Check sheet for the modelled part. Datum: model origin and axes. Units: mm. A direction names the side the tool comes from. Give positions to 0.01 mm unless a question says otherwise; leave off trailing zeros. Use a Markdown table: item, result. Add a question column.
1. Gauge pin test, flat ends, axial feed: P1, Ø4, axis at x = -4.195, z = 1.04, coming from the -Y side; P2, Ø0.5, axis at x = 4, z = 1, coming from the -Y side; P3, Ø0.5, axis at x = -4, z = 1, coming from the -Y side. Record the tip position at first contact, or that the pin passes through.
2. Release check for a two-part mould opening along X. For faces 1 (the cylindrical face through (-8.565, 6.83, 5.449)), 2 (the flat face through (0, 7, -5.75)), 3 (the flat face through (4, 4, 1)) record: released by +X, released by -X, zero draft, split by the parting line, or undercut.
3. Cross-section at A-A (y = 1.5). Count the separate pieces of the cut face and the enclosed holes in it, then the cut area to 3 significant figures.
4. Scan lines: probe 1 along X at (y, z) = (0.8, 1.04) (3 decimals); probe 2 along X at (y, z) = (0.5, 1.04) (3 decimals); probe 3 along Y at (x, z) = (4.5, 0.75). Record each from-to range of solid material in increasing order. Write a range as [from, to].
5. Set-up check for faces 4 (the cylindrical face through (2.21, 0.99, -0.48)), 5 (the cylindrical face through (-8.565, 0.301, 0.067)): record each of +Z, -Z, +X, -X, +Y, -Y from which the full face is reachable in a straight line by a thin tool's end or side.
Autodesk Fusion 360 part; units mm, degrees
sketch "Boceto1" plane through (0, 0, 0) normal (0, 1, 0) x (1, 0, 0)
  line L0 (-8.85, 0) -> (-8.85, -5.75)
  line L1 (-8.85, -5.75) -> (8.85, -5.75)
  line L2 (8.85, -5.75) -> (8.85, 5.75)
  line L3 (8.85, 5.75) -> (-8.85, 5.75)
  line L4 (-8.85, 5.75) -> (-8.85, 0)
  dimension "d1" = 8.85
  dimension "d2" = 5.75
  dimension "d3" = 17.7
  dimension "d4" = 11.5
  dimension "d5" = 17.7
extrude "Extruir1" add sketch "Boceto1" along normal blind 12.5
sketch "Boceto2" plane through (0, 0, 0) normal (0, -1, 0) x (1, 0, 0)
  line L0 (-8.85, 5.75) -> (-8.85, -5.75)
  line L1 (-8.85, -5.75) -> (8.85, -5.75)
  line L2 (8.85, -5.75) -> (8.85, 5.75)
  line L3 (8.85, 5.75) -> (-8.85, 5.75)
  line L4 (8.85, -5.75) -> (4.195, -5.75)
  line L5 (4.195, -5.75) -> (-4.195, -5.75)
  line L6 (4.195, -5.75) -> (4.195, 1.04)
  line L7 (-4.195, -5.75) -> (-4.195, 1.04)
  circle A0 centre (4.195, 1.04) radius 2.5
  circle A1 centre (-4.195, 1.04) radius 2.5
  dimension "d8" = 4.655
  dimension "d9" = 8.39
  dimension "d10" = 6.79
  dimension "d11" = 6.79
  dimension "d12" = 5
  dimension "d13" = 5
extrude "Extruir2" cut sketch "Boceto2" against normal blind 7 contours A0
extrude "Extruir3" cut sketch "Boceto2" against normal blind 7 contours A1
fillet "Empalme1" radius 1 3 edges at (8.85, 6.25, 5.75) (0, 0, 5.75) (8.85, 0, 0)
fillet "Empalme2" radius 1 3 edges at (-8.85, 0, -0.5) (-8.85, 0.2929, 5.4571) (-8.85, 6.75, 5.75)
fillet "Empalme3" radius 1 5 edges at (8.85, 6.75, -5.75) (8.5571, 0.2929, -5.75) (0, 0, -5.75) (-8.5571, 0.2929, -5.75) (-8.85, 6.75, -5.75)
extrude "Extruir4" add 1 faces at (4.9913, 7, -0.2658) along direction (0, -1, 0) blind 3
extrude "Extruir5" add 1 faces at (-4.4262, 7, 0.3911) along direction (0, -1, 0) blind 4
fillet "Empalme4" radius 2 1 faces at (4.9913, 4, -0.2658)
fillet "Empalme5" radius 2 1 faces at (-4.4262, 3, 0.3911)
Worked answers:
| question | item | result |
|---|---|---|
| 1 | P1 | stops at y = 2.32 |
| 1 | P2 | stops at y = 4 |
| 1 | P3 | stops at y = 3 |
| 2 | face 1 | released by -X |
| 2 | face 2 | zero draft |
| 2 | face 3 | undercut |
| 3 | separate pieces | 1 |
| 3 | enclosed holes | 2 |
| 3 | area | 164 mm² |
| 4 | probe 1 | x = [-8.83, -6.695], [-1.695, 1.695], [6.695, 8.83] |
| 4 | probe 2 | x = [-8.716, -6.695], [-1.695, 1.695], [6.695, 8.716] |
| 4 | probe 3 | y = [4, 12.5] |
| 5 | face 4 | -Y |
| 5 | face 5 | +Z, -Z, -X, -Y |
